Can you work these out from the model? Positions are in its coordinate system, mm. A direction names the side the tool comes from. Give positions to 0.01 mm unless a question says otherwise; leave off trailing zeros. Order: outer loops, then holes, each group sorted by start corner. A loop starts at its lowest first (then second) coordinate and runs counter-clockwise, first axis right, second up.
Item 1: I want a section at B-B, the plane x = 487. Write out the boundary of the cut face in (y, z) (3 decimals).
Item 2: If we mould it in two halves opening along Z, with no side actions, what happens to faces 1 (the flat face through (-7, 14, 34.925)), 2 (the flat face through (-7, 14, 38.1)), 3 (the flat face through (7, 14, -38.1)), 4 (the flat face through (7, 14, -34.925))? For each: +Z half, -Z half, draft (parallel to the pull), parting line (faces both ways), or undercut.
Item 3: If I drill on line 1 along X through (y, z) = (-2.35, 0); line 2 along Z through (x, y) = (-370, 17) (3 decimals); line 3 along Z through (x, y) = (317.5, -2.3), over which ranges is the centre line in solid material (lowest first)?
Item 4: I want a section at A-A, the plane y = 9.5. Write out the boundary of the cut face in (x, z) (3 decimals).
Item 5: I'm going to push flat-ended pins straight in: pin 1 Ø4 at (x, z) = (-146.05, -54.356) entering from +Y; pin 2 Ø1 at (x, y) = (558.5, -2.5) entering from +Z; pin 3 Ø10 at (y, z) = (6, 39) entering from +X; pin 4 Ø6.5 at (x, y) = (-47, 14) entering from +Z. Where does each tip first touch, or does it pass through?
Item 6: Which directions (+Z, -Z, +X, -X, +Y, -Y) give clear straight access to the entire face, cutting with the end or side of a thin tool? Please do faces 5 (the flat face through (-7, 27.432, 53)), 6 (the flat face through (8, 0, 0)), 7 (the flat face through (-520.7, 16.1, 37.6)), 8 (the flat face through (520.7, 16.1, 37.6)).
```python
from build123d import *

# Parameters (mm, degrees)
BASE_FLANGE2_DEPTH                     = 3.175
EDGE_FLANGE1_STRIP_W                   = 19.05
EDGE_FLANGE1_STRIP_H                   = 3.175
EDGE_FLANGE1_STRIP_CUT_DEPTH           = 1041.4
EDGE_FLANGE1_STRIP_2_W                 = 19.05
EDGE_FLANGE1_STRIP_2_H                 = 3.175
EDGE_FLANGE1_STRIP_CUT_2_DEPTH         = 1041.4
EDGE_FLANGE1_DEPTH                     = 1041.4
EDGE_FLANGE1_BEND_DEPTH                = 1041.4
EDGE_FLANGE3_START                     = -520.7
EDGE_FLANGE3_DEPTH                     = 1041.4
F_10_0_1935_DIAMETER_HOLE1_D           = 4.9149
F_10_0_1935_DIAMETER_HOLE1_ON_FACE_2_D = 4.9149
F_10_0_1935_DIAMETER_HOLE1_ON_FACE_3_D = 4.9149
F_17_64_0_26563_DIAMETER_HOLE1_D       = 6.747002
FILLET1_R                              = 3.175


# Read off the part's stored shape, not the designer's step: Edge-Flange3
# Sheet-metal steps are written as plain solids
with BuildPart() as part:
    # Sketch1 → Base-Flange2 (new body)
    with BuildSketch(Plane(origin=(0, 0, 0), x_dir=(1, 0, 0), z_dir=(0, 1, 0))):
        with BuildLine():
            Line((-520.7, 28.575), (-520.7, 38.1))
            Line((-520.7, 38.1), (520.7, 38.1))
            Line((520.7, 38.1), (520.7, 28.575))
            ThreePointArc((520.7, 28.575), (521.62993597, 26.32993597), (523.875, 25.4))
            Line((523.875, 25.4), (590.7405, 25.4))
            Line((590.7405, 25.4), (590.7405, -25.4))
            Line((590.7405, -25.4), (523.875, -25.4))
            ThreePointArc((523.875, -25.4), (521.62993597, -26.32993597), (520.7, -28.575))
            Line((520.7, -28.575), (520.7, -38.1))
            Line((520.7, -38.1), (-520.7, -38.1))
            Line((-520.7, -38.1), (-520.7, -28.575))
            ThreePointArc((-520.7, -28.575), (-521.62993597, -26.32993597), (-523.875, -25.4))
            Line((-523.875, -25.4), (-590.7405, -25.4))
            Line((-590.7405, -25.4), (-590.7405, 25.4))
            Line((-590.7405, 25.4), (-523.875, 25.4))
            ThreePointArc((-523.875, 25.4), (-521.62993597, 26.32993597), (-520.7, 28.575))
        make_face()
    extrude(amount=-BASE_FLANGE2_DEPTH)

    # Edge-Flange1 strip (across the edge) → Edge-Flange1 strip cut (cut)
    with BuildSketch(Plane(origin=(-520.7, 0, 38.1), x_dir=(0, 0, -1), z_dir=(1, 0, 0))):
        with Locations((-3.175, -1.5875)):
            Rectangle(EDGE_FLANGE1_STRIP_W, EDGE_FLANGE1_STRIP_H)
    extrude(amount=EDGE_FLANGE1_STRIP_CUT_DEPTH, mode=Mode.SUBTRACT)

    # Edge-Flange1 strip 2 (across the edge) → Edge-Flange1 strip cut 2 (cut)
    with BuildSketch(Plane(origin=(520.7, 0, -38.1), x_dir=(0, 0, 1), z_dir=(-1, 0, 0))):
        with Locations((-3.175, -1.5875)):
            Rectangle(EDGE_FLANGE1_STRIP_2_W, EDGE_FLANGE1_STRIP_2_H)
    extrude(amount=EDGE_FLANGE1_STRIP_CUT_2_DEPTH, mode=Mode.SUBTRACT)

    # Edge-Flange1 section (across the edge) → Edge-Flange1 (add)
    with BuildSketch(Plane(origin=(-520.7, 0, 38.1), x_dir=(0, 0, -1), z_dir=(1, 0, 0))):
        with BuildLine():
            Line((0, 3.175), (0, 17.145))
            Line((0, 17.145), (3.175, 17.145))
            Line((3.175, 17.145), (3.175, 3.175))
            ThreePointArc((3.175, 3.175), (4.10493597, 0.92993597), (6.35, 0))
            Line((6.35, 0), (6.35, -3.175))
            ThreePointArc((6.35, -3.175), (1.859871939, -1.315128061), (0, 3.175))
        make_face()
    extrude(amount=EDGE_FLANGE1_DEPTH)

    # Edge-Flange1 section 2 (across the edge) → Edge-Flange1 bend (add)
    with BuildSketch(Plane(origin=(520.7, 0, -38.1), x_dir=(0, 0, 1), z_dir=(-1, 0, 0))):
        with BuildLine():
            Line((0, 3.175), (0, 17.145))
            Line((0, 17.145), (3.175, 17.145))
            Line((3.175, 17.145), (3.175, 3.175))
            ThreePointArc((3.175, 3.175), (4.10493597, 0.92993597), (6.35, 0))
            Line((6.35, 0), (6.35, -3.175))
            ThreePointArc((6.35, -3.175), (1.859871939, -1.315128061), (0, 3.175))
        make_face()
    extrude(amount=EDGE_FLANGE1_BEND_DEPTH)

    # Edge-Flange3 outline → Edge-Flange3 (add)
    with BuildSketch(Plane.YZ.offset(EDGE_FLANGE3_START)):
        with BuildLine():
            Line((24.257, 38.1), (17.145, 38.1))
            Line((17.145, 38.1), (17.145, 34.925))
            Line((17.145, 34.925), (24.257, 34.925))
            ThreePointArc((24.257, 34.925), (28.747128061, 36.784871939), (30.607, 41.275))
            Line((30.607, 41.275), (30.607, 64.135))
            Line((30.607, 64.135), (27.432, 64.135))
            Line((27.432, 64.135), (27.432, 41.275))
            ThreePointArc((27.432, 41.275), (26.50206403, 39.02993597), (24.257, 38.1))
        make_face()
        with BuildLine():
            Line((17.145, -38.1), (24.257, -38.1))
            ThreePointArc((24.257, -38.1), (26.50206403, -39.02993597), (27.432, -41.275))
            Line((27.432, -41.275), (27.432, -64.135))
            Line((27.432, -64.135), (30.607, -64.135))
            Line((30.607, -64.135), (30.607, -41.275))
            ThreePointArc((30.607, -41.275), (28.747128061, -36.784871939), (24.257, -34.925))
            Line((24.257, -34.925), (17.145, -34.925))
            Line((17.145, -34.925), (17.145, -38.1))
        make_face()
    extrude(amount=EDGE_FLANGE3_DEPTH)

    # #10 (0.1935) Diameter Hole1 (through all)
    with Locations(Plane(origin=(-317.5, -3.175, 0), x_dir=(0, 0, -1), z_dir=(0, -1, 0))):
        with Locations((0, 0), (0, 635), (0, 317.5)):
            Hole(F_10_0_1935_DIAMETER_HOLE1_D / 2)

    # #10 (0.1935) Diameter Hole1 on face 2 (through all)
    with Locations(Plane.ZX):
        with Locations((0, 0)):
            Hole(F_10_0_1935_DIAMETER_HOLE1_ON_FACE_2_D / 2)

    # #10 (0.1935) Diameter Hole1 on face 3 (through all)
    with Locations(Plane(origin=(-438.15, 30.607, -54.356), x_dir=(0, 0, 1), z_dir=(0, 1, 0))):
        with Locations((0, 0), (0, 292.1), (0, 584.2), (0, 876.3), (108.712, 0), (108.712, 292.1), (108.712, 584.2), (108.712, 876.3)):
            Hole(F_10_0_1935_DIAMETER_HOLE1_ON_FACE_3_D / 2)

    # 17/64 (0.26563) Diameter Hole1 (through all)
    with Locations(Plane(origin=(-563.5625, 0, -12.7), x_dir=(0, 0, 1), z_dir=(0, 1, 0))):
        with Locations((0, 0), (25.4, 0), (0, 1127.125), (25.4, 1127.125)):
            Hole(F_17_64_0_26563_DIAMETER_HOLE1_D / 2)

    # Fillet1
    fillet1_edges = [part.edges().sort_by_distance(p)[0] for p in [
        (520.7, 29.0195, 64.135),
        (-520.7, 29.0195, 64.135),
        (-520.7, 29.0195, -64.135),
        (520.7, 29.0195, -64.135),
        (590.7405, -1.5875, -25.4),
        (590.7405, -1.5875, 25.4),
        (-590.7405, -1.5875, 25.4),
        (-590.7405, -1.5875, -25.4),
    ]]
    fillet(fillet1_edges, radius=FILLET1_R)


solid = part.part
```
Results list:
1. outline: (-3.175, -31.75) arc R6.35 ccw to (3.175, -38.1) - (24.257, -38.1) arc R3.175 cw to (27.432, -41.275) - (27.432, -64.135) - (30.607, -64.135) - (30.607, -41.275) arc R6.35 ccw to (24.257, -34.925) - (3.175, -34.925) arc R3.175 cw to (0, -31.75) - (0, 31.75) arc R3.175 cw to (3.175, 34.925) - (24.257, 34.925) arc R6.35 ccw to (30.607, 41.275) - (30.607, 64.135) - (27.432, 64.135) - (27.432, 41.275) arc R3.175 cw to (24.257, 38.1) - (3.175, 38.1) arc R6.35 ccw to (-3.175, 31.75) - close
2. face 1: undercut
2. face 2: +Z half
2. face 3: -Z half
2. face 4: undercut
3. line 1: x = -590.74 to -319.96, -315.04 to -2.46, 2.46 to 315.04, 319.96 to 590.74
3. line 2: z = -38.1 to -34.925, 34.925 to 38.1
3. line 3: z = -34.97 to -2.46, 2.46 to 34.97
4. outline: (-520.7, -38.1) - (520.7, -38.1) - (520.7, -34.925) - (-520.7, -34.925) - close; (-520.7, 34.925) - (520.7, 34.925) - (520.7, 38.1) - (-520.7, 38.1) - close
5. pin 1: passes through
5. pin 2: stops at z = 25.4
5. pin 3: stops at x = 520.7
5. pin 4: stops at z = 38.1
6. face 5: +Z, +X, -X, -Y
6. face 6: +X, -X, +Y
6. face 7: +Z, -X, +Y, -Y
6. face 8: +Z, +X, +Y, -Y
